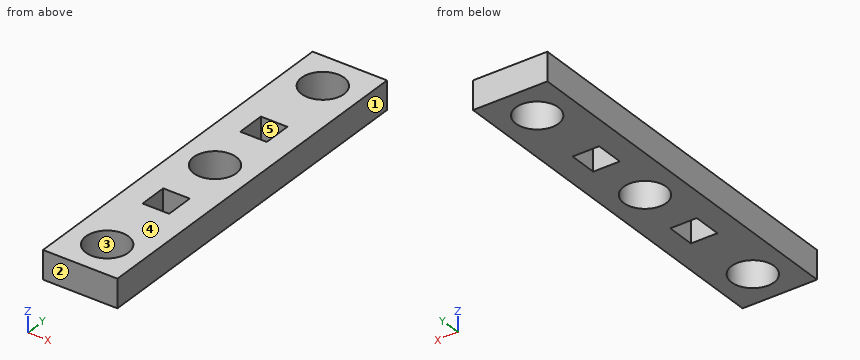
```python
from build123d import *

# Parameters (mm, degrees)
MODEL_W             = 14
MODEL_H             = 70
MODEL_R             = 4
MODEL_W_2           = 5
MODEL_H_2           = 5.35
BOSS_EXTRUDE1_DEPTH = 5.35


with BuildPart() as part:
    # Model → Boss-Extrude1 (new body)
    with BuildSketch(Plane.XY):
        with Locations((7, 35)):
            Rectangle(MODEL_W, MODEL_H)
        with Locations((7, 63)):
            Circle(MODEL_R, mode=Mode.SUBTRACT)
        with Locations(Location((7, 7, 0), (0, 0, 180))):
            Circle(MODEL_R, mode=Mode.SUBTRACT)
        with Locations((7, 35)):
            Circle(MODEL_R, mode=Mode.SUBTRACT)
        with Locations((7, 47.675)):
            Rectangle(MODEL_W_2, MODEL_H_2, mode=Mode.SUBTRACT)
        with Locations((7, 22.325)):
            Rectangle(MODEL_W_2, MODEL_H_2, mode=Mode.SUBTRACT)
    extrude(amount=BOSS_EXTRUDE1_DEPTH)


solid = part.part
```
Part model, mm, in its own coordinate system. Face numbers are marked on the shaded views. A direction names the side the tool comes from. Round coordinates to 2 decimals unless told otherwise and drop trailing zeros. Write each loop counter-clockwise with the first axis right and the second up, starting at its lowest first coordinate (ties: lowest second). Pieces come first, ordered by that corner, then holes. Notation, with made-up numbers: M 66.25,-13.5 L 96.25,-13.5 A9 ccw 96.25,2.5 Z; hole C 10.25,24 d4. An arc over 180 degrees is marked long. One line per question, with ' | ' between items.
(1) Probe line 1 along Y through (x, z) = (7, 1.7); line 2 along Y through (x, z) = (6.25, 0.5). List the from-to ranges inside material, lowest first.
Answer key:
line 1: y = 0 to 3, 11 to 19.65, 25 to 31, 39 to 45, 50.35 to 59, 67 to 70 | line 2: y = 0 to 3.07, 10.93 to 19.65, 25 to 31.07, 38.93 to 45, 50.35 to 59.07, 66.93 to 70
(2) Saw through at C-C on x = 7. Write the cut outline in (y, z), then the cut area to 3 significant figures.
Answer key:
outline: M 0,0 L 3,0 L 3,5.35 L 0,5.35 Z; M 11,0 L 19.65,0 L 19.65,5.35 L 11,5.35 Z; M 25,0 L 31,0 L 31,5.35 L 25,5.35 Z; M 39,0 L 45,0 L 45,5.35 L 39,5.35 Z; M 50.35,0 L 59,0 L 59,5.35 L 50.35,5.35 Z; M 67,0 L 70,0 L 70,5.35 L 67,5.35 Z | area: 189 mm^2
(3) Saw through at A-A on y = 7. Write the cut outline in (x, z), then the cut area to 3 significant figures.
Answer key:
outline: M 0,0 L 3,0 L 3,5.35 L 0,5.35 Z; M 11,0 L 14,0 L 14,5.35 L 11,5.35 Z | area: 32.1 mm^2
(4) 3-axis set-ups, long thin cutter, end or side, ignore diameter. For the marked faces 4 and 5: which of +Z, -Z, +X, -X, +Y, -Y reach the whole face in a straight line?
Answer key:
face 4: +Z, +X, -X, +Y, -Y | face 5: +Z, -Z
(5) Pin check, flat tips, straight feed: pin 1 (1.5 mm diameter, centred on x = 7.5, z = 2.5, fed in from -Y); pin 2 (5 mm diameter, centred on x = 7, y = 7, fed in from -Z). Stop position of each tip, or through.
Answer key:
pin 1: stops at y = 0 | pin 2: passes through
(6) Saw through at D-D on y = 37. Write the cut outline in (x, z), then the cut area to 3 significant figures.
Answer key:
outline: M 0,0 L 3.54,0 L 3.54,5.35 L 0,5.35 Z; M 10.46,0 L 14,0 L 14,5.35 L 10.46,5.35 Z | area: 37.8 mm^2
(7) Saw through at B-B on z = 3.8. Write the cut outline in (x, y), then the cut area to 3 significant figures.
Answer key:
outline: M 0,0 L 14,0 L 14,70 L 0,70 Z; hole C 7,7 d8; hole C 7,35 d8; hole C 7,63 d8; hole M 4.5,19.65 L 9.5,19.65 L 9.5,25 L 4.5,25 Z; hole M 4.5,45 L 9.5,45 L 9.5,50.35 L 4.5,50.35 Z | area: 776 mm^2
(8) Two-plate mould, pull along X, no slides. Class the marked faces 1, 2 and 3: released by +X, released by -X, zero draft, split by the parting line, or undercut.
Answer key:
face 1: released by +X | face 2: zero draft | face 3: undercut
